```python
from build123d import *

# Parameters (mm, degrees)
SKETCH3_R               = 1.25
BOSS_EXTRUDE2_DEPTH     = 0.8
CUT_EXTRUDE1_DEPTH      = 1.8
CUT_EXTRUDE1_DEPTH_BACK = 1.8
FILLET1_R               = 4


with BuildPart() as part:
    # Sketch3 → Boss-Extrude2 (new body, symmetric)
    with BuildSketch(Plane(origin=(0, 0, 0), x_dir=(1, 0, 0), z_dir=(0, 1, 0))):
        with BuildLine():
            Line((-41.16248371, 28.383973204), (-19.371710273, 15.803064294))
            ThreePointArc((-19.371710273, 15.803064294), (-21.650635095, -12.5), (4, -24.677925359))
            Line((4, -24.677925359), (4, -49.839743178))
            ThreePointArc((4, -49.839743178), (-43.301270189, -25), (-41.16248371, 28.383973204))
        make_face()
        with Locations((-32.475952642, 18.75)):
            Circle(SKETCH3_R, mode=Mode.SUBTRACT)
        with Locations((0, -37.5)):
            Circle(SKETCH3_R, mode=Mode.SUBTRACT)
    extrude(amount=BOSS_EXTRUDE2_DEPTH, both=True)

    # Sketch4 → Cut-Extrude1 (cut, two sides)
    with BuildSketch(Plane(origin=(0, 0, 0), x_dir=(1, 0, 0), z_dir=(0, 1, 0))) as cut_extrude1_sk:
        Polygon((-24.132543601, -34.736441086), (-15.303067673, -39.431156714), (-18.589368612, -45.611789864), (-27.418844541, -40.917074236), align=None)
        Polygon((-39.431156714, -15.303067673), (-34.736441086, -24.132543601), (-40.917074236, -27.418844541), (-45.611789864, -18.589368612), align=None)
        Polygon((-40.554257724, -11.550527282), (-37.866498102, -18.55238048), (-44.401561088, -21.060956127), (-47.089320709, -14.059102928), align=None)
        Polygon((-42.293315139, -0.524875766), (-40.988053217, -10.43932438), (-47.928167246, -11.353007726), (-49.233429168, -1.438559112), align=None)
    extrude(amount=CUT_EXTRUDE1_DEPTH, mode=Mode.SUBTRACT)
    extrude(cut_extrude1_sk.sketch, amount=-CUT_EXTRUDE1_DEPTH_BACK, mode=Mode.SUBTRACT)

    # Fillet1
    fillet1_edges = [part.edges().sort_by_distance(p)[0] for p in [
        (-41.16248371, 0, -28.383973204),
        (-19.371710273, 0, -15.803064294),
        (4, 0, 24.677925359),
        (4, 0, 49.839743178),
    ]]
    fillet(fillet1_edges, radius=FILLET1_R)


solid = part.part
```
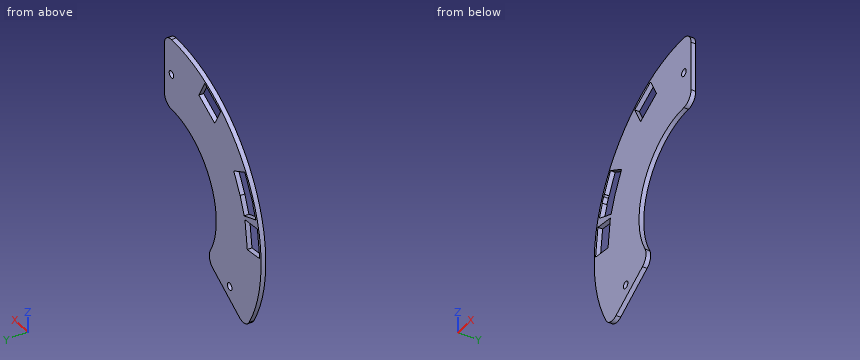
Verification items for the finished model (mm, model axes). Coordinates: 2 decimals unless noted, no trailing zeros. Loops run counter-clockwise (first coordinate to the right, second up) from the corner with the lowest first, then second, coordinate; pieces in that order, holes last. Notation, with made-up numbers: (-12.75, 71.5) -> (5.25, 71.5) arc R15 cw to (5.25, 79.5) -> close; hole circle Ø10 at (83, 2.25). An arc over 180 degrees is marked (long way). Answer in a Markdown table with one row per item. Add a question column.
1. Section check D-D, the plane z = 37.5. Enter the section's corners in (x, y).
2. Material ranges on probe 1 along Z at (x, y) = (0, -0.4); probe 2 along X at (y, z) = (-0.1, 37.5); probe 3 along Z at (x, y) = (-42.5, 0.15), recorded low to high. Write a range as [from, to].
3. Section check C-C, the plane y = -0.25. Enter the section's corners in (x, z), then the cut area to 3 significant figures.
4. Section check B-B, the plane z = -18.75. Enter the section's corners in (x, y), then the cut area to 3 significant figures.
5. Section check A-A, the plane x = -32.5. Enter the section's corners in (y, z), then the cut area to 3 significant figures.
Derived:
| question | item | result |
|---|---|---|
| 1 | outline | (-33.07, -0.8) -> (-25.6, -0.8) -> (-25.6, 0.8) -> (-33.07, 0.8) -> close; (-18.94, -0.8) -> (-1.25, -0.8) -> (-1.25, 0.8) -> (-18.94, 0.8) -> close; (1.25, -0.8) -> (4, -0.8) -> (4, 0.8) -> (1.25, 0.8) -> close |
| 2 | probe 1 | z = [25, 36.25], [38.75, 50] |
| 2 | probe 2 | x = [-33.07, -25.6], [-18.94, -1.25], [1.25, 4] |
| 2 | probe 3 | z = [-25.98, 0.55], [10.64, 12.3], [24.44, 26.34] |
| 3 | outline | (-43.3, -25) arc R4 ccw to (-37.84, -26.46) -> (-23.11, -17.96) arc R4 ccw to (-21.65, -12.5) arc R25 cw to (0, 25) arc R4 ccw to (4, 29) -> (4, 46) arc R4 ccw to (0, 50) arc R50 ccw to start; hole (-49.23, 1.44) -> (-42.29, 0.52) -> (-40.99, 10.44) -> (-47.93, 11.35) -> close; hole (-47.09, 14.06) -> (-40.55, 11.55) -> (-38.29, 17.45) -> (-34.74, 24.13) -> (-40.92, 27.42) -> (-44.32, 21.03) -> (-44.4, 21.06) -> (-44.67, 20.36) -> (-45.61, 18.59) -> (-45.39, 18.47) -> close; hole circle Ø2.5 at (-32.48, -18.75); hole (-27.42, 40.92) -> (-24.13, 34.74) -> (-15.3, 39.43) -> (-18.59, 45.61) -> close; hole circle Ø2.5 at (0, 37.5) |
| 3 | area | 1,900 mm² |
| 4 | outline | (-46.35, -0.8) -> (-33.73, -0.8) -> (-33.73, 0.8) -> (-46.35, 0.8) -> close; (-31.23, -0.8) -> (-24.48, -0.8) -> (-24.48, 0.8) -> (-31.23, 0.8) -> close |
| 4 | area | 31.0 mm² |
| 5 | outline | (-0.8, -23.38) -> (0.8, -23.38) -> (0.8, -20) -> (-0.8, -20) -> close; (-0.8, -17.5) -> (0.8, -17.5) -> (0.8, 38) -> (-0.8, 38) -> close |
| 5 | area | 94.2 mm² |
